Read the model definition and answer for the solid it produces. Units are mm, in the model's axes. Give positions to 0.01 mm unless a question says otherwise; leave off trailing zeros. Loops run counter-clockwise (first coordinate to the right, second up) from the corner with the lowest first, then second, coordinate; pieces in that order, holes last. Notation, with made-up numbers: (9, 37) -> (37, 37) arc R14 ccw to (37, 63) -> close; hole circle Ø1 at (88, -22). An arc over 180 degrees is marked (long way). Write each question's results on one line, items separated by ' | '. Start each with the question number.
Item 1: Determine the mould class of faces 1 (the flat face through (-4.5, 16.4, -6.35)), 2 (the cylindrical face through (-3.648, -16.427, 0.089)), 3 (the conical face through (-16.031, -12.292, -5.953)) for opening direction Y: +Y half, -Y half, draft (parallel to the pull), parting line (faces both ways), or undercut.
Item 2: Each of these flat-tipped pins is pushed along its axis until it touches: P1, Ø1.5, axis at y = -2, z = -3.5, coming from the +X side; P2, Ø6, axis at y = 2, z = -5, coming from the +X side; P3, Ø4, axis at y = 8, z = 3, coming from the -X side. Where does it stop, or does it pass through?
Item 3: Section C-C on z = 2.5 is taken. Write down the section's boundary in (x, y) (1 decimal), and give its area (3 significant figures).
Item 4: Section B-B on z = -3.5 is taken. Write down the section's boundary in (x, y) (1 decimal), and give its area (3 significant figures).
Item 5: Find the intervals of material crossed by line 1 (Y direction, x = -12, z = 4); line 2 (Y direction, x = 6, z = -5.5); line 3 (X direction, y = -2.5, z = 4.25), in increasing order.
Item 6: Section A-A on x = 0 is taken. Write down the section's boundary in (y, z), and give its area (3 significant figures).
```python
from build123d import *

# Parameters (mm, degrees)
F0_R     = 20.0025
F0_R_2   = 16.8275
F1_DEPTH = 6.35
F3_R     = 20.0025
F2_R     = 23.1775
F6_R     = 16.8275
F7_DEPTH = 12.701


with BuildPart() as f1:
    # F0 (on Top) → F1 (new body)
    with BuildSketch(Plane.XY):
        Circle(F0_R)
        Circle(F0_R_2, mode=Mode.SUBTRACT)
    extrude(amount=F1_DEPTH)

    # F3 (on face) → F4 section 0
    with BuildSketch(Plane.XY.offset(6.35)):
        Circle(F3_R)
    # F2 (on Top) → F4 section 1
    with BuildSketch(Plane.XY):
        Circle(F2_R)
    loft()

    # F5: F1 across plane


with BuildPart() as f1_1:
    add(f1.part)
    add(f1.part.mirror(Plane.XY))

    # F6 (on face) → F7 (cut, through all)
    with BuildSketch(Plane.XY.offset(6.35)):
        Circle(F6_R)
    extrude(amount=-F7_DEPTH, mode=Mode.SUBTRACT)


solid = f1_1.part
```
Findings:
1) face 1: draft | face 2: undercut | face 3: parting line
2) P1: x = 21.72 | P2: x = 22.11 | P3: x = -21.43
3) outline: circle Ø43.9 at (0, 0); hole circle Ø33.7 at (0, 0) | area: 621 mm2
4) outline: circle Ø42.9 at (0, 0); hole circle Ø33.7 at (0, 0) | area: 553 mm2
5) line 1: -17.45 to -11.8, 11.8 to 17.45 | line 2: -19.53 to -15.72, 15.72 to 19.53 | line 3: -20.9 to -16.64, 16.64 to 20.9
6) outline: (-23.18, 0) -> (-20, -6.35) -> (-16.83, -6.35) -> (-16.83, 6.35) -> (-20, 6.35) -> close; (16.83, -6.35) -> (20, -6.35) -> (23.18, 0) -> (20, 6.35) -> (16.83, 6.35) -> close | area: 121 mm2
